from build123d import *

# Parameters (mm, degrees)
CROQUIS2_W              = 40
CROQUIS2_H              = 55
CROQUIS2_R              = 2
SALIENTE_EXTRUIR1_DEPTH = 2
CROQUIS3_W              = 40
CROQUIS3_H              = 2
SALIENTE_EXTRUIR2_DEPTH = 42
CROQUIS4_R              = 4
SALIENTE_EXTRUIR3_DEPTH = 2
MATRIZL1_COUNT          = 2
MATRIZL1_PITCH          = 12
CROQUIS6_W              = 40
CROQUIS6_H              = 15
CORTAR_EXTRUIR1_DEPTH   = 10


with BuildPart() as part:
    # Croquis2 → Saliente-Extruir1 (new body)
    with BuildSketch(Plane(origin=(0, 0, 0), x_dir=(1, 0, 0), z_dir=(0, 1, 0))):
        with Locations((20, 27.5)):
            Rectangle(CROQUIS2_W, CROQUIS2_H)
        with Locations(Location((5, 47.5, 0), (0, 0, 270))):
            Circle(CROQUIS2_R, mode=Mode.SUBTRACT)
        with Locations(Location((35, 47.5, 0), (0, 0, 270))):
            Circle(CROQUIS2_R, mode=Mode.SUBTRACT)
        with Locations(Location((35, 7.5, 0), (0, 0, 270))):
            Circle(CROQUIS2_R, mode=Mode.SUBTRACT)
        with Locations(Location((5, 7.5, 0), (0, 0, 270))):
            Circle(CROQUIS2_R, mode=Mode.SUBTRACT)
    extrude(amount=SALIENTE_EXTRUIR1_DEPTH)

    # Croquis3 → Saliente-Extruir2 (add)
    with BuildSketch(Plane(origin=(0, 0, 0), x_dir=(1, 0, 0), z_dir=(0, 1, 0))):
        with Locations((20, -1)):
            Rectangle(CROQUIS3_W, CROQUIS3_H)
    extrude(amount=SALIENTE_EXTRUIR2_DEPTH)

    # Croquis4 → Saliente-Extruir3 (add)
    with BuildSketch(Plane(origin=(0, 22, 0), x_dir=(1, 0, 0), z_dir=(0, 1, 0))):
        with BuildLine():
            Line((40, 15), (40, 0))
            Line((40, 0), (21, 0))
            Line((21, 0), (21, 15))
            ThreePointArc((21, 15), (30.5, 24.5), (40, 15))
        make_face()
        with Locations(Location((30.5, 15, 0), (0, 0, 270))):
            Circle(CROQUIS4_R, mode=Mode.SUBTRACT)
    saliente_extruir3 = extrude(amount=SALIENTE_EXTRUIR3_DEPTH)

    # MatrizL1: Saliente-Extruir3 ×2
    with Locations(*[(0, -i * MATRIZL1_PITCH, 0) for i in range(1, MATRIZL1_COUNT)]):
        add(saliente_extruir3)

    # Croquis6 → Cortar-Extruir1 (cut)
    with BuildSketch(Plane(origin=(0, 0, 0), x_dir=(-1, 0, 0), z_dir=(0, 0, -1))):
        with Locations((-20, 34.5)):
            Rectangle(CROQUIS6_W, CROQUIS6_H)
    extrude(amount=-CORTAR_EXTRUIR1_DEPTH, mode=Mode.SUBTRACT)


solid = part.part
CAD build for the part. Positions are in the model's coordinates, mm. A direction names the side the tool comes from. Round coordinates to 2 decimals unless told otherwise and drop trailing zeros. Loops run counter-clockwise (first coordinate to the right, second up) from the corner with the lowest first, then second, coordinate; pieces in that order, holes last.
(1) Two-plate mould, pull along X, no slides. Class faces 1 (the cylindrical face through (30.291, 22.986, -24.498)), 2 (the cylindrical face through (34.466, 22.986, -15.521)), 3 (the flat face through (21, 23, -7)): +X half, -X half, draft (parallel to the pull), parting line (faces both ways), or undercut.
(2) Cut at A-A (z = -4). Give the cut face in (x, y), plus the area to 3 significant figures.
(3) Drop flat-ended pins along their axis: pin 1 (8 mm diameter, centred on y = 16, z = -29.5, fed in from -X); pin 2 (1 mm diameter, centred on y = 10.5, z = -11, fed in from -X); pin 3 (5 mm diameter, centred on x = 29.5, z = -28, fed in from +Y); pin 4 (6 mm diameter, centred on x = 25, y = 9, fed in from -Z). Give the stop position or say it passes through.
(4) Wall check: line 1 along X through (y, z) = (0.75, -47.5); line 2 along Y through (x, z) = (31, -21); line 3 along X through (y, z) = (22.6, -15). Give the ranges that are in metal, low to high.
(5) Cut at D-D (x = 5). Give the cut face in (y, z).
(6) Cut at C-C (y = 23). Give the cut face in (x, z).
(7) Which spindle directions (+Z, -Z, +X, -X, +Y, -Y) get a long thin tool onto all of the face, cutting with end or side? Do faces 4 (the cylindrical face through (34.466, 10.986, -15.521)), 5 (the flat face through (31, 10, -10)), 6 (the flat face through (20, 14, 0)). Say none if no direction does.
(8) Cut at B-B (x = 30.5). Give the cut face in (y, z), plus the area to 3 significant figures.
Findings below:
1. face 1: parting line
1. face 2: undercut
1. face 3: -X half
2. outline: (0, 0) - (40, 0) - (40, 2) - (0, 2) - close; (21, 10) - (40, 10) - (40, 12) - (21, 12) - close; (21, 22) - (40, 22) - (40, 24) - (21, 24) - close
2. area: 156 mm2
3. pin 1: passes through
3. pin 2: stops at x = 21
3. pin 3: stops at y = 2
3. pin 4: stops at z = -24.12
4. line 1: x = 0 to 3, 7 to 33, 37 to 40
4. line 2: y = 0 to 2, 10 to 12, 22 to 24
4. line 3: x = 21 to 26.5, 34.5 to 40
5. outline: (0, -55) - (2, -55) - (2, -49.5) - (0, -49.5) - close; (0, -45.5) - (2, -45.5) - (2, -9.5) - (0, -9.5) - close; (0, -5.5) - (2, -5.5) - (2, 0) - (27, 0) - (27, 2) - (0, 2) - close
6. outline: (0, 0) - (21, 0) - (21, -15) arc R9.5 ccw to (40, -15) - (40, 2) - (0, 2) - close; hole circle Ø8 at (30.5, -15)
7. face 4: +Y
7. face 5: -Z, +X, -X
7. face 6: -Z, -X
8. outline: (0, -55) - (2, -55) - (2, 0) - (10, 0) - (10, -11) - (12, -11) - (12, 0) - (22, 0) - (22, -11) - (24, -11) - (24, 0) - (27, 0) - (27, 2) - (0, 2) - close; (10, -24.5) - (12, -24.5) - (12, -19) - (10, -19) - close; (22, -24.5) - (24, -24.5) - (24, -19) - (22, -19) - close
8. area: 230 mm2
